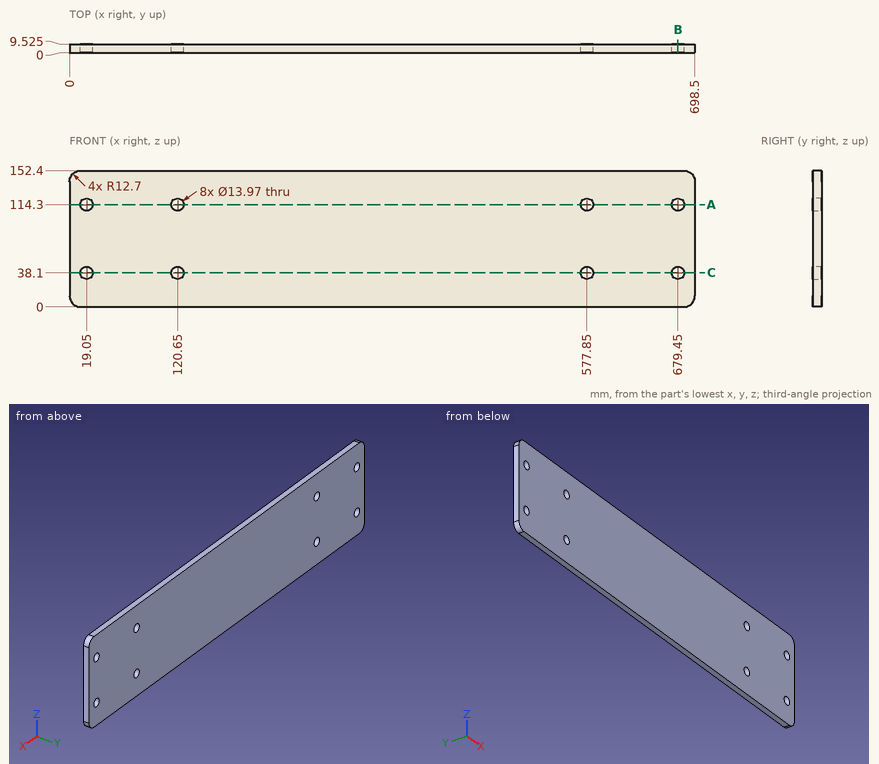
Check sheet for the drawn part. Datum: minimum x, y, z corner. Units: mm. Round coordinates to 2 decimals unless told otherwise and drop trailing zeros. Order: outer loops, then holes, each group sorted by start corner. A loop starts at its lowest first (then second) coordinate and runs counter-clockwise, first axis right, second up.
(1) Cross-section at B-B, the plane x = 679.45. Enter the section's corners in (y, z) (3 decimals).
(2) Cross-section at C-C, the plane z = 38.5. Enter the section's corners in (x, y) (3 decimals), and give its area (3 significant figures).
(3) Cross-section at A-A, the plane z = 114.3. Enter the section's corners in (x, y) (3 decimals).
(4) Scan lines: probe 1 along X at (y, z) = (5.5, 38.1) (3 decimals); probe 2 along Z at (x, y) = (120.65, 2) (3 decimals); probe 3 along Z at (x, y) = (116.5, 0.5). Record each from-to range of solid material in increasing order.
Check sheet entries:
1. outline: (0, 0) - (9.525, 0) - (9.525, 31.115) - (0, 31.115) - close; (0, 45.085) - (9.525, 45.085) - (9.525, 107.315) - (0, 107.315) - close; (0, 121.285) - (9.525, 121.285) - (9.525, 152.4) - (0, 152.4) - close
2. outline: (0, 0) - (12.076, 0) - (12.076, 9.525) - (0, 9.525) - close; (26.024, 0) - (113.676, 0) - (113.676, 9.525) - (26.024, 9.525) - close; (127.624, 0) - (570.876, 0) - (570.876, 9.525) - (127.624, 9.525) - close; (584.824, 0) - (672.476, 0) - (672.476, 9.525) - (584.824, 9.525) - close; (686.424, 0) - (698.5, 0) - (698.5, 9.525) - (686.424, 9.525) - close
2. area: 6,120 mm2
3. outline: (0, 0) - (12.065, 0) - (12.065, 9.525) - (0, 9.525) - close; (26.035, 0) - (113.665, 0) - (113.665, 9.525) - (26.035, 9.525) - close; (127.635, 0) - (570.865, 0) - (570.865, 9.525) - (127.635, 9.525) - close; (584.835, 0) - (672.465, 0) - (672.465, 9.525) - (584.835, 9.525) - close; (686.435, 0) - (698.5, 0) - (698.5, 9.525) - (686.435, 9.525) - close
4. probe 1: x = 0 to 12.065, 26.035 to 113.665, 127.635 to 570.865, 584.835 to 672.465, 686.435 to 698.5
4. probe 2: z = 0 to 31.115, 45.085 to 107.315, 121.285 to 152.4
4. probe 3: z = 0 to 32.48, 43.72 to 108.68, 119.92 to 152.4
